Autodesk Inventor part; units mm, degrees
ref_plane "YZ Plane" through (0, 0, 0) normal (1, 0, 0) x (0, 1, 0)
ref_plane "XZ Plane" through (0, 0, 0) normal (0, 1, 0) x (-1, 0, 0)
ref_plane "XY Plane" through (0, 0, 0) normal (0, 0, 1) x (1, 0, 0)
sketch "Sketch1" plane through (0, 0, 0) normal (0, 1, 0) x (-1, 0, 0)
  circle A0 centre (0, 0) radius 6.5
  line L0 (0, 6.5) -> (15, 6.5)
  line L1 (15, 6.5) -> (15, -6.5)
  line L2 (15, -6.5) -> (0, -6.5)
  line L3 (0, -6.5) -> (0, 6.5)
  line L4 (15, 2.5) -> (85, 2.5)
  line L5 (85, 2.5) -> (85, -2.5)
  line L6 (85, -2.5) -> (15, -2.5)
  line L7 (15, -2.5) -> (15, 2.5)
  dimension "d0" = 13
  dimension "d1" = 6.5
  dimension "d2" = 15
  dimension "d3" = 6.5
  dimension "d4" = 70
  dimension "d5" = 4
  dimension "d6" = 4
extrude "Extrusion1" add sketch "Sketch1" along normal blind 4
fillet "Fillet1" radius 2 2 edges at (-50, 4, -2.5) (-50, 0, -2.5)
sketch "Sketch2" plane through (-85, 0, 2.5) normal (0, 0, 1) x (1, 0, 0)
  line L0 (70, 0) -> (70, 4)
  line L1 (0, 4) -> (70, 4)
  line L2 (70, 0) -> (65, 0)
  line L3 (65, 0) -> (65, 4)
  line L4 (65, 4) -> (70, 4)
  line L5 (70, 4) -> (70, 0)
  point P0 (85, 0)
  dimension "d10" = 5
extrude "Extrusion2" add sketch "Sketch2" along normal blind 15
properties part number "Arms"
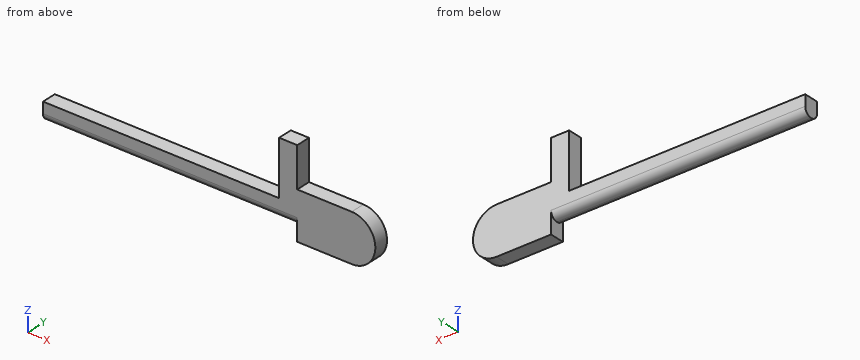
Geometry check sheet. Reference: the model listing, model coordinates, mm. Round coordinates to 2 decimals unless told otherwise and drop trailing zeros. Write each loop counter-clockwise with the first axis right and the second up, starting at its lowest first coordinate (ties: lowest second). Pieces come first, ordered by that corner, then holes.
Item 1: Material ranges on line 1 along Z through (x, y) = (-8, 2.8); line 2 along Z through (x, y) = (-41, 2.1); line 3 along X through (y, z) = (2.4, 0.5), recorded low to high.
Determined:
line 1: z = -6.5 to 6.5
line 2: z = -2.5 to 2.5
line 3: x = -85 to 6.48
Item 2: Section check A-A (y = 3). Record the boundary of the cut face in (x, z).
Determined:
outline: (-85, -2.23) - (-15, -2.23) - (-15, -6.5) - (0, -6.5) arc R6.5 ccw to (0, 6.5) - (-15, 6.5) - (-15, 17.5) - (-20, 17.5) - (-20, 2.5) - (-85, 2.5) - close
Item 3: Section check D-D (x = -3.5). Record the boundary of the cut face in (y, z), plus the area to 3 significant figures.
Determined:
outline: (0, -6.5) - (4, -6.5) - (4, 6.5) - (0, 6.5) - close
area: 52.0 mm2
Item 4: Section check C-C (z = 16.25). Record the boundary of the cut face in (x, y), plus the area to 3 significant figures.
Determined:
outline: (-20, 0) - (-15, 0) - (-15, 4) - (-20, 4) - close
area: 20.0 mm2
Item 5: Go/stop test with flat-tipped pins: pin 1 Ø1.2 at (x, y) = (-4, 2) entering from +Z; pin 2 Ø2 at (y, z) = (2, 12) entering from +X; pin 3 Ø1.5 at (x, z) = (-34.5, 3.5) entering from +Y; pin 4 Ø1.5 at (y, z) = (3.5, 9.5) entering from -X. Record where each tip stops, or that it passes through.
Determined:
pin 1: stops at z = 6.5
pin 2: stops at x = -15
pin 3: passes through
pin 4: stops at x = -20
